```python
from build123d import *

# Parameters (mm, degrees)
SKETCH1_W           = 80
SKETCH1_H           = 10
BOSS_EXTRUDE1_DEPTH = 40
SKETCH2_R           = 47.5
CUT_EXTRUDE1_DEPTH  = 7.5
SKETCH3_R           = 50
CUT_EXTRUDE2_DEPTH  = 6.5
FILLET1_R           = 2
FILLET2_R           = 2


with BuildPart() as part:
    # Sketch1 → Boss-Extrude1 (new body)
    with BuildSketch(Plane(origin=(0, 0, 0), x_dir=(1, 0, 0), z_dir=(0, 1, 0))):
        with Locations((-2.66565113, -7.064446738)):
            Rectangle(SKETCH1_W, SKETCH1_H)
    extrude(amount=BOSS_EXTRUDE1_DEPTH)

    # Sketch2 → Cut-Extrude1 (cut)
    with BuildSketch(Plane.XY.offset(12.064446738)):
        with Locations((-3.625057346, 50.093821186)):
            Circle(SKETCH2_R)
    extrude(amount=-CUT_EXTRUDE1_DEPTH, mode=Mode.SUBTRACT)

    # Sketch3 → Cut-Extrude2 (cut)
    with BuildSketch(Plane.XY.offset(11.064446738)):
        with Locations((-3.625057346, 50.093821186)):
            Circle(SKETCH3_R)
    extrude(amount=-CUT_EXTRUDE2_DEPTH, mode=Mode.SUBTRACT)

    # Fillet1
    fillet1_edges = [part.edges().sort_by_distance(p)[0] for p in [
        (-42.66565113, 40, 3.314446738),
        (37.33434887, 40, 3.314446738),
    ]]
    fillet(fillet1_edges, radius=FILLET1_R)

    # Fillet2
    fillet2_edges = [part.edges().sort_by_distance(p)[0] for p in [
        (-2.66565113, 40, 2.064446738),
        (-42.66565113, 19, 2.064446738),
        (37.33434887, 19, 2.064446738),
        (-42.079864693, 39.414213562, 2.064446738),
        (36.748562432, 39.414213562, 2.064446738),
    ]]
    fillet(fillet2_edges, radius=FILLET2_R)


solid = part.part
```
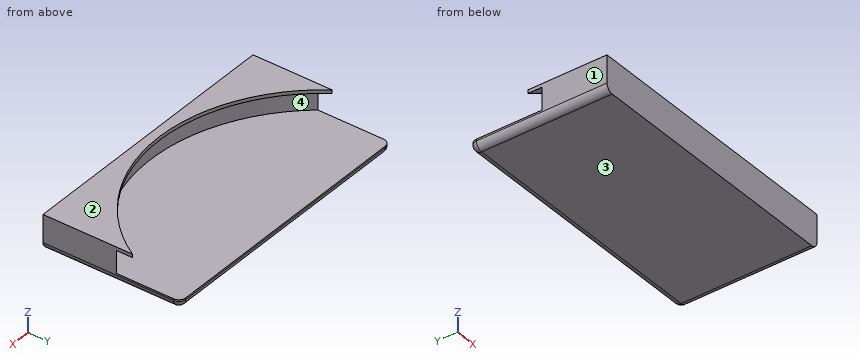
For this review, take the finished solid that the model builds, in its own axes (mm). Face numbers are marked on the shaded views. Round coordinates to 2 decimals unless told otherwise and drop trailing zeros. Write each loop counter-clockwise with the first axis right and the second up, starting at its lowest first coordinate (ties: lowest second). Pieces come first, ordered by that corner, then holes. Notation, with made-up numbers: (87, 49) -> (111, 49) arc R27 cw to (111, 71) -> close; hole circle Ø10 at (59.25, 49.25). An arc over 180 degrees is marked (long way). One line per question, with ' | ' between items. Start each with the question number.
(1) Insertion check: P1, Ø2, axis at y = 24.5, z = 10, coming from the -X side; P2, Ø8, axis at x = 2.5, y = 32.5, coming from the +Z side. Each pin has a flat end and moves straight along its axis. Give the tip position at first contact, or say it passes through.
(2) Add section A-A, the plane y = 20.5. Write out the cut boundary in (x, z), plus the area to 3 significant figures.
(3) Add section C-C, the plane y = 13. Write out the cut boundary in (x, z).
(4) For line 1 along Z through (x, y) = (1, 19.5); line 2 along X through (y, z) = (15, 8); line 3 along X through (y, z) = (18.5, 6.5), list the stretches that pass through material, from the lowest coordinate up. Write a range as from..to.
(5) Mouldability with a two-part tool opening along Z and no side actions: class the marked faces 1, 2, 3 and 4 as released by +Z, released by -Z, zero draft, split by the parting line, or undercut.
(6) Add section B-B, the plane x = 23.5. Write out the cut boundary in (y, z), plus the area to 3 significant figures.
(7) Add section D-D, the plane x = -13.5. Write out the cut boundary in (y, z).
Answer list:
1) P1: through | P2: z = 4.56
2) outline: (-42.67, 4.06) arc R2 ccw to (-40.67, 2.06) -> (35.33, 2.06) arc R2 ccw to (37.33, 4.06) -> (37.33, 12.06) -> (33.53, 12.06) -> (33.53, 11.06) -> (36.68, 11.06) -> (36.68, 4.56) -> (-42.67, 4.56) -> close; (-42.67, 11.06) -> (-40.78, 11.06) -> (-40.78, 12.06) -> (-42.67, 12.06) -> close | area: 208 mm²
3) outline: (-42.67, 4.06) arc R2 ccw to (-40.67, 2.06) -> (35.33, 2.06) arc R2 ccw to (37.33, 4.06) -> (37.33, 12.06) -> (26.04, 12.06) -> (26.04, 11.06) -> (29.9, 11.06) -> (29.9, 4.56) -> (-37.15, 4.56) -> (-37.15, 11.06) -> (-33.29, 11.06) -> (-33.29, 12.06) -> (-42.67, 12.06) -> close
4) line 1: 2.06..4.56 | line 2: -42.67..-39.24, 31.99..37.33 | line 3: -42.67..-42.38, 35.13..37.33
5) face 1: zero draft | face 2: released by +Z | face 3: released by -Z | face 4: undercut
6) outline: (0, 2.06) -> (38, 2.06) arc R2 ccw to (40, 4.06) -> (40, 4.56) -> (8.09, 4.56) -> (8.09, 11.06) -> (11.1, 11.06) -> (11.1, 12.06) -> (0, 12.06) -> close | area: 163 mm²
7) outline: (0, 2.06) -> (38, 2.06) arc R2 ccw to (40, 4.06) -> (40, 4.56) -> (1.08, 4.56) -> (1.08, 11.06) -> (3.63, 11.06) -> (3.63, 12.06) -> (0, 12.06) -> close
